Check sheet for the drawn part. Datum: minimum x, y, z corner. Units: mm. A direction names the side the tool comes from. Coordinates: 2 decimals unless noted, no trailing zeros. Order: outer loops, then holes, each group sorted by start corner. A loop starts at its lowest first (then second) coordinate and runs counter-clockwise, first axis right, second up. Notation, with made-up numbers: (-3, 59.25) -> (50, 59.25) arc R30 cw to (50, 98.25) -> close; hole circle Ø2 at (-12.75, -17.5). An arc over 180 degrees is marked (long way). Answer as CSV lines item,"result".
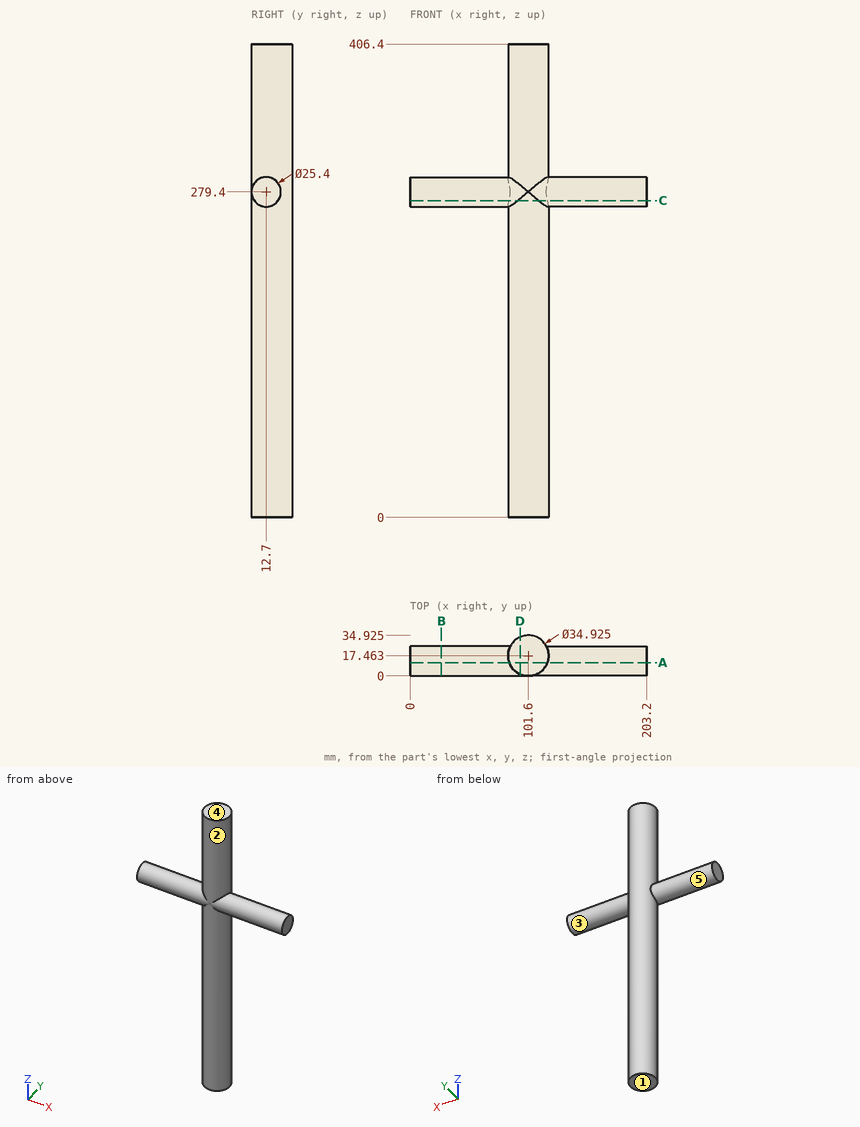
Item 1: Depth check by flat-ended pin: pin 1 Ø12 at (x, y) = (167.5, 21.5) entering from -Z; pin 2 Ø8 at (x, y) = (27, 15.5) entering from +Z; pin 3 Ø3 at (y, z) = (17.5, 53.5) entering from -X. Enter the tip coordinate at first touch or a pass-through.
Answer list:
pin 1,"z = 267.01"
pin 2,"z = 292.1"
pin 3,"x = 84.14"
Item 2: Section check A-A, the plane y = 11.5. Record the boundary of the cut face in (x, z).
Answer list:
outline,"(0, 266.76) -> (85.19, 266.76) -> (85.19, 0) -> (118.01, 0) -> (118.01, 266.76) -> (203.2, 266.76) -> (203.2, 292.04) -> (118.01, 292.04) -> (118.01, 406.4) -> (85.19, 406.4) -> (85.19, 292.04) -> (0, 292.04) -> close"
Item 3: Section check C-C, the plane z = 272. Record the boundary of the cut face in (x, y) (1 decimal).
Answer list:
outline,"(0, 2.4) -> (92.8, 2.4) arc R17.5 ccw to (110.4, 2.4) -> (203.2, 2.4) -> (203.2, 23) -> (118.2, 23) arc R17.5 ccw to (85, 23) -> (0, 23) -> close"
Item 4: Section check D-D, the plane x = 94.5. Record the boundary of the cut face in (y, z).
Answer list:
outline,"(1.51, 0) -> (33.42, 0) -> (33.42, 406.4) -> (1.51, 406.4) -> (1.51, 285.4) arc R12.7 ccw to (1.51, 273.4) -> close"
Item 5: Tool access check on the marked faces 1, 2, 3, 4 and 5. Record the directions out of +Z, -Z, +X, -X, +Y, -Y that give a thin tool (end or side, any length) a straight path to the whole face; none if there is none.
Answer list:
face 1,"-Z, +X, -X, +Y, -Y"
face 2,"none"
face 3,"+X"
face 4,"+Z, +X, -X, +Y, -Y"
face 5,"-X"
Item 6: Thickness scan on line 1 (Y direction, x = 102, z = 66) (1 decimal); line 2 (Z direction, x = 18, y = 20); line 3 (X direction, y = 16, z = 244). Record the ranges inside material, lowest first.
Answer list:
line 1,"0 to 34.9"
line 2,"269.01 to 289.79"
line 3,"84.2 to 119"
Item 7: Section check B-B, the plane x = 27. Record the boundary of the cut face in (y, z), plus the area to 3 significant figures.
Answer list:
outline,"circle Ø25.4 at (12.7, 279.4)"
area,"507 mm2"
